Geometry check sheet. Reference: drawing and pictorial views, mm from the part's lowest x, y, z. A direction names the side the tool comes from. Give positions to 0.01 mm unless a question says otherwise; leave off trailing zeros. Write each loop counter-clockwise with the first axis right and the second up, starting at its lowest first coordinate (ties: lowest second). Pieces come first, ordered by that corner, then holes. Notation, with made-up numbers: (63, -7.75) -> (106, -7.75) arc R15 ccw to (106, 5.25) -> close; hole circle Ø6 at (75.25, 46.25). An arc over 180 degrees is marked (long way). Return JSON: item names as keys, results as strings.
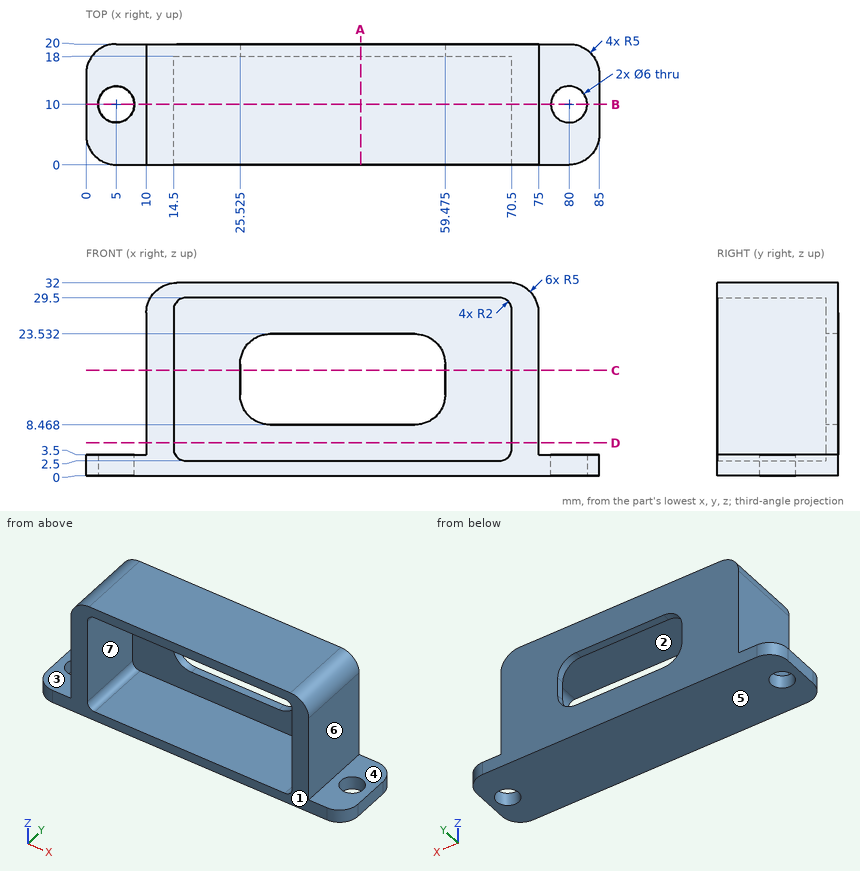
(1) Cross-section at B-B on y = 10. Enter the section's corners in (x, z), then the cut area to 3 significant figures.
Reply:
{"outline": "(0, 0) -> (2, 0) -> (2, 3.5) -> (0, 3.5) -> close; (8, 0) -> (77, 0) -> (77, 3.5) -> (75, 3.5) -> (75, 27) arc R5 ccw to (70, 32) -> (15, 32) arc R5 ccw to (10, 27) -> (10, 3.5) -> (8, 3.5) -> close; (83, 0) -> (85, 0) -> (85, 3.5) -> (83, 3.5) -> close; hole (14.5, 4.5) arc R2 ccw to (16.5, 2.5) -> (68.5, 2.5) arc R2 ccw to (70.5, 4.5) -> (70.5, 27.5) arc R2 ccw to (68.5, 29.5) -> (16.5, 29.5) arc R2 ccw to (14.5, 27.5) -> close", "area": "589 mm^2"}
(2) Release check for a two-part mould opening along X. For the marked faces 5, 6 and 7 record: pulls with the +X half, pulls with the -X half, needs draft (parallel to the pull), parting line crosses it, or undercut.
Reply:
{"face 5": "needs draft", "face 6": "pulls with the +X half", "face 7": "undercut"}
(3) Cross-section at C-C on z = 17.5. Enter the section's corners in (x, y) (1 decimal).
Reply:
{"outline": "(10, 0) -> (14.5, 0) -> (14.5, 18) -> (25.5, 18) -> (25.5, 20) -> (10, 20) -> close; (59.5, 18) -> (70.5, 18) -> (70.5, 0) -> (75, 0) -> (75, 20) -> (59.5, 20) -> close"}
(4) Depth check by flat-ended pin: pin 1 Ø2 at (y, z) = (17, 17.5) entering from +X; pin 2 Ø1 at (x, z) = (32, 8.5) entering from -Y; pin 3 Ø5 at (y, z) = (11.5, 12) entering from -X. Enter the tip coordinate at first touch or a pass-through.
Reply:
{"pin 1": "x = 75", "pin 2": "y = 18", "pin 3": "x = 10"}
(5) Thickness scan on L1, parallel to Z at x = 32.5, y = 14.75; L2, parallel to Y at x = 80, z = 1.4; L3, parallel to X at y = 2, z = 25.5. Record the ranges inside material, lowest first.
Reply:
{"L1": "0 to 2.5, 29.5 to 32", "L2": "0 to 7, 13 to 20", "L3": "10 to 14.5, 70.5 to 75"}
(6) Cross-section at A-A on x = 45.5. Enter the section's corners in (y, z), then the cut area to 3 significant figures.
Reply:
{"outline": "(0, 0) -> (20, 0) -> (20, 8.47) -> (18, 8.47) -> (18, 2.5) -> (0, 2.5) -> close; (0, 29.5) -> (18, 29.5) -> (18, 23.53) -> (20, 23.53) -> (20, 32) -> (0, 32) -> close", "area": "124 mm^2"}
(7) Set-up check for the marked faces 1, 2, 3 and 4: record each of +Z, -Z, +X, -X, +Y, -Y from which the full face is reachable in a straight line by a thin tool's end or side.
Reply:
{"face 1": "+Z, -Z, +X, -X, -Y", "face 2": "-Y", "face 3": "+Z, -X, +Y, -Y", "face 4": "+Z, +X, +Y, -Y"}
(8) Cross-section at D-D on z = 5.5. Enter the section's corners in (x, y), then the cut area to 3 significant figures.
Reply:
{"outline": "(10, 0) -> (14.5, 0) -> (14.5, 18) -> (70.5, 18) -> (70.5, 0) -> (75, 0) -> (75, 20) -> (10, 20) -> close", "area": "292 mm^2"}
